from build123d import *

# Parameters (mm, degrees)
F0_R     = 6.386329
F0_R_2   = 7.669861
F1_DEPTH = 76.2


with BuildPart() as f1:
    # F0 (on Front) → F1 (new body)
    with BuildSketch(Plane.XZ):
        with BuildLine():
            Line((-59.575226, -25.464874), (-59.575226, -46.214029))
            Line((-59.575226, -46.214029), (0, -46.214029))
            Line((0, -46.214029), (0, -14.775913))
            Line((0, -14.775913), (-10.846913, -14.775913))
            Line((-10.846913, -14.775913), (-51.715698, -14.775913))
            ThreePointArc((-51.715698, -14.775913), (-57.398857, -18.831133), (-59.575226, -25.464874))
        make_face()
        with Locations((-25.837737, -32.445498)):
            Circle(F0_R, mode=Mode.SUBTRACT)
        with BuildLine():
            Line((-67.434758, -46.214029), (-59.575226, -46.214029))
            Line((-59.575226, -46.214029), (-59.575226, -25.464874))
            ThreePointArc((-59.575226, -25.464874), (-57.398857, -18.831133), (-51.715698, -14.775913))
            Line((-51.715698, -14.775913), (-10.846913, -14.775913))
            Line((-10.846913, -14.775913), (-10.846913, -9.121778))
            Line((-10.846913, -9.121778), (-57.374559, -9.121778))
            ThreePointArc((-57.374559, -9.121778), (-64.731001, -16.236777), (-67.434758, -26.107447))
            Line((-67.434758, -26.107447), (-67.434758, -46.214029))
        make_face()
        Polygon((-10.846913, -14.775913), (0, -14.775913), (9.588626, -14.775913), (21.832943, -26.408015), (44.932198, -17.93753), (44.932198, 22.635443), (12.734826, 42.775784), (-10.846913, 50.652135), (-10.846913, -9.121778), align=None)
        with Locations((16.108637, 8.963856)):
            Circle(F0_R_2, mode=Mode.SUBTRACT)
        with BuildLine():
            Line((0, -14.775913), (0, -46.214029))
            Line((0, -46.214029), (20.277588, -46.214029))
            ThreePointArc((20.277588, -46.214029), (31.173466, -45.250121), (41.730902, -42.388338))
            ThreePointArc((41.730902, -42.388338), (37.981593, -41.004981), (34.739118, -38.668882))
            Line((34.739118, -38.668882), (30.417925, -34.563749))
            Line((30.417925, -34.563749), (21.832943, -26.408015))
            Line((21.832943, -26.408015), (9.588626, -14.775913))
            Line((9.588626, -14.775913), (0, -14.775913))
        make_face()
        with BuildLine():
            ThreePointArc((34.739118, -38.668882), (37.981593, -41.004981), (41.730902, -42.388338))
            ThreePointArc((41.730902, -42.388338), (50.726835, -38.231397), (58.946468, -32.69564))
            Line((58.946468, -32.69564), (52.658845, -26.408015))
            Line((52.658845, -26.408015), (52.602403, -26.428712))
            Line((52.602403, -26.428712), (30.417925, -34.563749))
            Line((30.417925, -34.563749), (34.739118, -38.668882))
        make_face()
        Polygon((44.932198, -17.93753), (21.832943, -26.408015), (30.417925, -34.563749), (52.602403, -26.428712), (51.715698, 22.635443), (44.932198, 22.635443), align=None)
        Polygon((21.853101, 50.320085), (12.734826, 42.775784), (44.932198, 22.635443), (51.715698, 22.635443), (54.86754, 30.485805), align=None)
        Polygon((0, 59.769187), (-10.846913, 50.652135), (12.734826, 42.775784), (21.853101, 50.320085), align=None)
    extrude(amount=F1_DEPTH)


solid = f1.part
Work out the finished part from the listing and answer in its coordinate system (mm). A direction names the side the tool comes from. Give positions to 0.01 mm unless a question says otherwise; leave off trailing zeros. Loops run counter-clockwise (first coordinate to the right, second up) from the corner with the lowest first, then second, coordinate; pieces in that order, holes last. Notation, with made-up numbers: (27.25, -15.5) -> (36.25, -15.5) arc R20 cw to (36.25, 5.5) -> close; hole circle Ø11 at (-11, -17). An arc over 180 degrees is marked (long way). Use a Markdown table: item, result. Add a question column.
1) The part is cut by section D-D, the plane z = -14. Determine the outline of the cut face in (x, y).
2) The part is cut by section C-C, the plane x = -51.5. Determine the outline of the cut face in (y, z), plus the area to 3 significant figures.
3) Which of the six approach directions +Z, -Z, +X, -X, +Y, -Y give full straight-line access (tool end or side, diameter ignored) to faces 1 (the flat face through (-67.435, -38, -36)), 2 (the flat face through (53.27, -37.57, 26.51)), 3 (the flat face through (-34, -38, -9.122))?
4) The part is cut by section B-B, the plane y = -6.5. Determine the outline of the cut face in (x, z).
5) The part is cut by section A-A, the plane z = -35. Determine the outline of the cut face in (x, y), plus the area to 3 significant figures.
6) For a pull along Z with two mould halves and no side action, classify faces 4 (the cylindrical face through (-64.657, -37.567, -16.112)), 5 (the flat face through (9, -76.2, -4)), 6 (the flat face through (55.85, -37.57, -29.6)) as +Z half, -Z half, draft (parallel to the pull), parting line (faces both ways), or undercut.
7) Consider line 1 along Z through (x, y) = (-24, -37); line 2 along Z through (x, y) = (-41.5, -50.5); line 3 along Z through (x, y) = (11, -34.5). Determine where each line is inside the solid, lowest interval first.
8) Each of these flat-tipped pins is pushed along its axis until it touches: P1, Ø2, axis at y = -45, z = 3, coming from the -X side; P2, Ø3, axis at y = -64, z = -24.5, coming from the +X side; P3, Ø14, axis at x = 16.11, z = 8.96, coming from the -Y side; P4, Ø1.5, axis at y = -41.5, z = -31.5, coming from the +X side. Where does it stop, or does it pass through?
Reported:
| question | item | result |
|---|---|---|
| 1 | outline | (-63.18, -76.2) -> (52.38, -76.2) -> (52.38, 0) -> (-63.18, 0) -> close |
| 2 | outline | (-76.2, -46.21) -> (0, -46.21) -> (0, -9.12) -> (-76.2, -9.12) -> close |
| 2 | area | 2,830 mm^2 |
| 3 | face 1 | +Z, -Z, -X, +Y, -Y |
| 3 | face 2 | +X, +Y, -Y |
| 3 | face 3 | +Z, -X, +Y, -Y |
| 4 | outline | (-67.43, -46.21) -> (20.28, -46.21) arc R62.06 ccw to (41.73, -42.39) arc R62.06 ccw to (58.95, -32.7) -> (52.66, -26.41) -> (52.6, -26.43) -> (51.72, 22.64) -> (54.87, 30.49) -> (21.85, 50.32) -> (0, 59.77) -> (-10.85, 50.65) -> (-10.85, -9.12) -> (-57.37, -9.12) arc R19.37 ccw to (-67.43, -26.11) -> close; hole circle Ø12.77 at (-25.84, -32.45); hole circle Ø15.34 at (16.11, 8.96) |
| 5 | outline | (-67.43, -76.2) -> (-31.69, -76.2) -> (-31.69, 0) -> (-67.43, 0) -> close; (-19.98, -76.2) -> (55.86, -76.2) -> (55.86, 0) -> (-19.98, 0) -> close |
| 5 | area | 8,500 mm^2 |
| 6 | face 4 | +Z half |
| 6 | face 5 | draft |
| 6 | face 6 | undercut |
| 7 | line 1 | z = -46.21 to -38.56, -26.33 to -9.12 |
| 7 | line 2 | z = -46.21 to -9.12 |
| 7 | line 3 | z = -46.21 to 3.24, 14.68 to 55.01 |
| 8 | P1 | stops at x = -10.85 |
| 8 | P2 | stops at x = 52.59 |
| 8 | P3 | passes through |
| 8 | P4 | stops at x = 58.5 |
